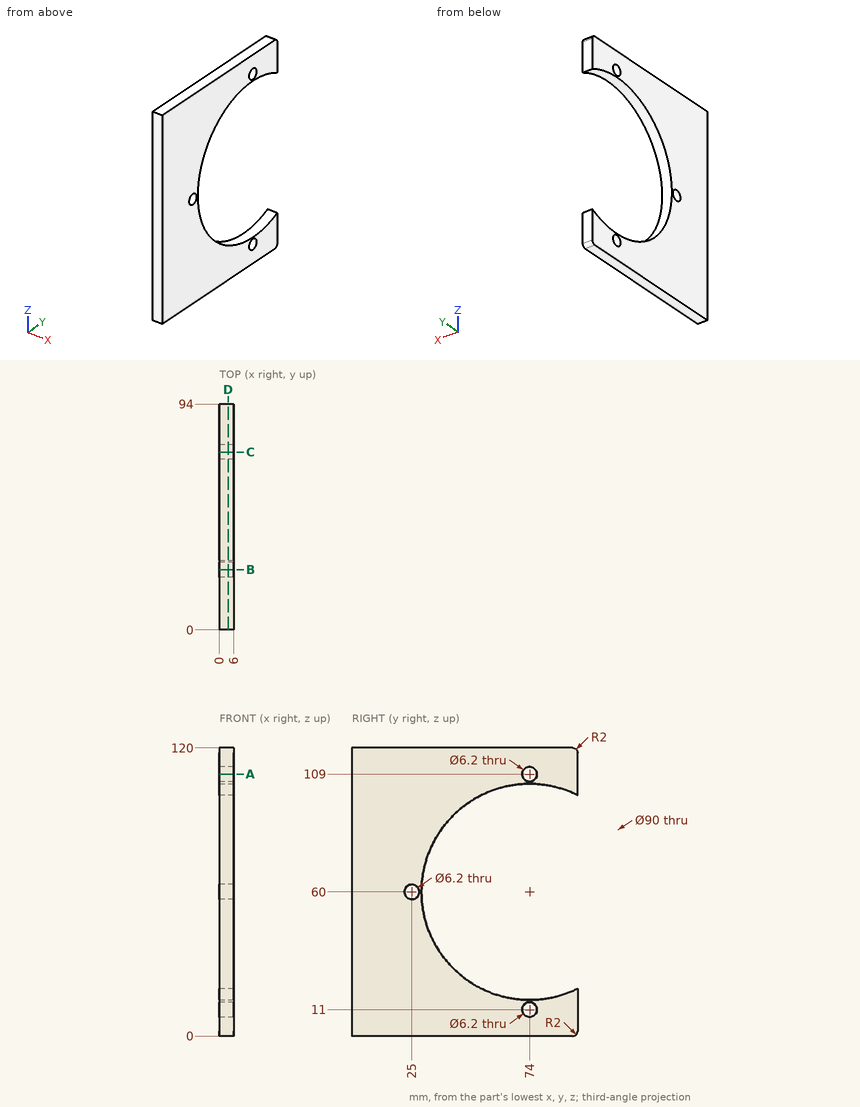
For this review, use the dimensioned drawing (mm, ordinates from the lowest corner) and the shaded views. Round coordinates to 2 decimals unless told otherwise and drop trailing zeros. Write each loop counter-clockwise with the first axis right and the second up, starting at its lowest first coordinate (ties: lowest second). Pieces come first, ordered by that corner, then holes. Notation, with made-up numbers: (-26.5, 51.25) -> (-4.5, 51.25) arc R26 cw to (-4.5, 82.25) -> close; hole circle Ø6 at (-15.5, 0.5). An arc over 180 degrees is marked (long way). Use CSV: the item, a comma, the result in double quotes.
(1) Consider section D-D, the plane x = 3.6. Give the boundary of the cut face in (y, z), plus the area to 3 significant figures.
Computed values:
outline,"(0, 0) -> (92, 0) arc R2 ccw to (94, 2) -> (94, 19.69) arc R45 cw (long way) to (94, 100.31) -> (94, 118) arc R2 ccw to (92, 120) -> (0, 120) -> close; hole circle Ø6.2 at (25, 60); hole circle Ø6.2 at (74, 11); hole circle Ø6.2 at (74, 109)"
area,"6,270 mm²"
(2) To check wall thickness, follow L1, parallel to Z at x = 2.6, y = 25; L2, parallel to Z at x = 3.05, y = 74; L3, parallel to Y at x = 2.25, z = 109. State the ranges of each line that lie inside material, in increasing order. Write a range as [from, to].
Computed values:
L1,"[0, 56.9], [63.1, 120]"
L2,"[0, 7.9], [14.1, 15], [105, 105.9], [112.1, 120]"
L3,"[0, 70.9], [77.1, 94]"
(3) Consider section A-A, the plane z = 109. Give the boundary of the cut face in (x, y), plus the area to 3 significant figures.
Computed values:
outline,"(0, 0) -> (6, 0) -> (6, 70.9) -> (0, 70.9) -> close; (0, 77.1) -> (6, 77.1) -> (6, 94) -> (0, 94) -> close"
area,"527 mm²"
(4) Consider section B-B, the plane y = 25. Give the boundary of the cut face in (x, z), plus the area to 3 significant figures.
Computed values:
outline,"(0, 0) -> (6, 0) -> (6, 56.9) -> (0, 56.9) -> close; (0, 63.1) -> (6, 63.1) -> (6, 120) -> (0, 120) -> close"
area,"683 mm²"
(5) Consider section C-C, the plane y = 74. Give the boundary of the cut face in (x, z).
Computed values:
outline,"(0, 0) -> (6, 0) -> (6, 7.9) -> (0, 7.9) -> close; (0, 14.1) -> (6, 14.1) -> (6, 15) -> (0, 15) -> close; (0, 105) -> (6, 105) -> (6, 105.9) -> (0, 105.9) -> close; (0, 112.1) -> (6, 112.1) -> (6, 120) -> (0, 120) -> close"
(6) Clearance check with flat-ended pins moving along their axes: P1, Ø1, axis at x = 4.5, z = 35.5, coming from the +Y side; P2, Ø8, axis at y = 79.5, z = 22.5, coming from the +X side. State where each tip first meets the part, or that it passes through.
Computed values:
P1,"y = 36.58"
P2,"through"
